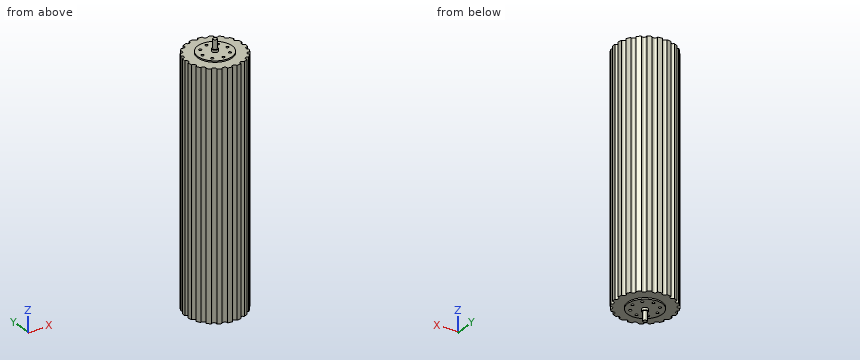
from build123d import *

# Parameters (mm, degrees)
SKETCH1_R               = 127
BOSS_EXTRUDE1_DEPTH     = 527
SKETCH4_R               = 12.5
BOSS_EXTRUDE3_DEPTH     = 584
BOSS_EXTRUDE4_START     = 6
SKETCH5_R               = 75
SKETCH5_R_2             = 12.5
BOSS_EXTRUDE4_DEPTH     = 6
CUT_EXTRUDE1_DEPTH      = 1132.347426744
CUT_EXTRUDE1_DEPTH_BACK = 1132.347426744
SKETCH6_R               = 6
CUT_EXTRUDE2_DEPTH      = 1126.42392013
CUT_EXTRUDE2_DEPTH_BACK = 1126.42392013
SKETCH7_R               = 10
SKETCH8_R               = 12.5
SKETCH8_R_2             = 8.5
CUT_EXTRUDE4_DEPTH      = 40
CUT_EXTRUDE5_START      = -40
SKETCH10_R              = 12.5
SKETCH10_R_2            = 8.5
CUT_EXTRUDE5_DEPTH      = 40


with BuildPart() as part:
    # Sketch1 → Boss-Extrude1 (new, symmetric)
    with BuildSketch(Plane.XY):
        Circle(SKETCH1_R)
    extrude(amount=BOSS_EXTRUDE1_DEPTH, both=True)

    # Sketch4 → Boss-Extrude3 (add, symmetric)
    with BuildSketch(Plane(origin=(0, 0, 0), x_dir=(-1, 0, 0), z_dir=(0, 0, -1))):
        with Locations(Location((0, 0, 0), (0, 0, 180))):
            Circle(SKETCH4_R)
    boss_extrude3 = extrude(amount=BOSS_EXTRUDE3_DEPTH, both=True)

    # Sketch5 → Boss-Extrude4 (add)
    with BuildSketch(Plane(origin=(0, 0, -527), x_dir=(-1, 0, 0), z_dir=(0, 0, -1)).offset(BOSS_EXTRUDE4_START)):
        with Locations(Location((0, 0, 0), (0, 0, 180))):
            Circle(SKETCH5_R)
        with Locations(Location((0, 0, 0), (0, 0, 180))):
            Circle(SKETCH5_R_2, mode=Mode.SUBTRACT)
    boss_extrude4 = extrude(amount=-BOSS_EXTRUDE4_DEPTH)

    # Mirror1: Boss-Extrude3, Boss-Extrude4 across plane
    add(boss_extrude3.mirror(Plane(origin=(0, 0, 0), x_dir=(1, 0, 0), z_dir=(0, 0, -1))))
    add(boss_extrude4.mirror(Plane(origin=(0, 0, 0), x_dir=(1, 0, 0), z_dir=(0, 0, -1))))

    # Sketch6 → Cut-Extrude1 (cut, two sides: drawn at the far end of the back side and taken through both)
    with BuildSketch(Plane(origin=(0, 0, -533), x_dir=(-1, 0, 0), z_dir=(0, 0, -1)).offset(-CUT_EXTRUDE1_DEPTH_BACK)):
        with Locations((0, 55)):
            Circle(SKETCH6_R)
        with Locations((38.890872965, 38.890872965)):
            Circle(SKETCH6_R)
        with Locations((55, 0)):
            Circle(SKETCH6_R)
        with Locations((38.890872965, -38.890872965)):
            Circle(SKETCH6_R)
        with Locations((0, -55)):
            Circle(SKETCH6_R)
        with Locations((-38.890872965, -38.890872965)):
            Circle(SKETCH6_R)
        with Locations((-55, 0)):
            Circle(SKETCH6_R)
        with Locations((-38.890872965, 38.890872965)):
            Circle(SKETCH6_R)
    extrude(amount=CUT_EXTRUDE1_DEPTH + CUT_EXTRUDE1_DEPTH_BACK, mode=Mode.SUBTRACT)

    # Sketch7 → Cut-Extrude2 (cut, two sides: drawn at the far end of the back side and taken through both)
    with BuildSketch(Plane(origin=(0, 0, -527), x_dir=(-1, 0, 0), z_dir=(0, 0, -1)).offset(-CUT_EXTRUDE2_DEPTH_BACK)):
        with Locations((0, 127)):
            Circle(SKETCH7_R)
        with Locations((39.245158286, 120.784177569)):
            Circle(SKETCH7_R)
        with Locations((74.648727041, 102.745158286)):
            Circle(SKETCH7_R)
        with Locations((102.745158286, 74.648727041)):
            Circle(SKETCH7_R)
        with Locations((120.784177569, 39.245158286)):
            Circle(SKETCH7_R)
        with Locations((127, 0)):
            Circle(SKETCH7_R)
        with Locations((120.784177569, -39.245158286)):
            Circle(SKETCH7_R)
        with Locations((102.745158286, -74.648727041)):
            Circle(SKETCH7_R)
        with Locations((74.648727041, -102.745158286)):
            Circle(SKETCH7_R)
        with Locations((39.245158286, -120.784177569)):
            Circle(SKETCH7_R)
        with Locations((0, -127)):
            Circle(SKETCH7_R)
        with Locations((-39.245158286, -120.784177569)):
            Circle(SKETCH7_R)
        with Locations((-74.648727041, -102.745158286)):
            Circle(SKETCH7_R)
        with Locations((-102.745158286, -74.648727041)):
            Circle(SKETCH7_R)
        with Locations((-120.784177569, -39.245158286)):
            Circle(SKETCH7_R)
        with Locations((-127, 0)):
            Circle(SKETCH7_R)
        with Locations((-120.784177569, 39.245158286)):
            Circle(SKETCH7_R)
        with Locations((-102.745158286, 74.648727041)):
            Circle(SKETCH7_R)
        with Locations((-74.648727041, 102.745158286)):
            Circle(SKETCH7_R)
        with Locations((-39.245158286, 120.784177569)):
            Circle(SKETCH7_R)
    extrude(amount=CUT_EXTRUDE2_DEPTH + CUT_EXTRUDE2_DEPTH_BACK, mode=Mode.SUBTRACT)

    # Sketch8 → Cut-Extrude4 (cut)
    with BuildSketch(Plane(origin=(0, 0, -584), x_dir=(-1, 0, 0), z_dir=(0, 0, -1))):
        Circle(SKETCH8_R)
        Circle(SKETCH8_R_2, mode=Mode.SUBTRACT)
    extrude(amount=-CUT_EXTRUDE4_DEPTH, mode=Mode.SUBTRACT)

    # Sketch10 → Cut-Extrude5 (cut)
    with BuildSketch(Plane.XY.offset(584).offset(CUT_EXTRUDE5_START)):
        Circle(SKETCH10_R)
        with Locations(Location((0, 0, 0), (0, 0, 180))):
            Circle(SKETCH10_R_2, mode=Mode.SUBTRACT)
    extrude(amount=CUT_EXTRUDE5_DEPTH, mode=Mode.SUBTRACT)


solid = part.part
Part model, mm, in its own coordinate system. Give positions to 0.01 mm unless a question says otherwise; leave off trailing zeros.
1) Pin check, flat tips, straight feed: pin 1 (14 mm diameter, centred on x = -38.89, y = -38.89, fed in from +Z); pin 2 (7 mm diameter, centred on x = 38.89, y = -38.89, fed in from +Z); pin 3 (2 mm diameter, centred on x = -31.5, z = 109, fed in from -Y); pin 4 (15.5 mm diameter, centred on x = 0, y = 55, fed in from -Z). Stop position of each tip, or through.
Resolved:
pin 1: stops at z = 533
pin 2: passes through
pin 3: stops at y = -115.93
pin 4: stops at z = -533
2) Probe L1, parallel to X at y = -39.5, z = 107.5; L2, parallel to Y at x = 0, z = -137; L3, parallel to Y at x = -1.5, z = 115.5. List the from-to ranges inside material, lowest first.
Resolved:
L1: x = -110.79 to -44.86, -32.92 to 32.92, 44.86 to 110.79
L2: y = -117 to -61, -49 to 49, 61 to 117
L3: y = -117.11 to -60.81, -49.19 to 49.19, 60.81 to 117.11
3) Cut at A-A on z = -209. State how many separate pieces and enclosed holes the cut face has, then the cut area to 3 significant figures.
Resolved:
separate pieces: 1
enclosed holes: 8
area: 46,700 mm2
